Here's how the part is built. I have some questions about the finished solid (model axes, mm). Give positions to 0.01 mm unless a question says otherwise; leave off trailing zeros. Loops run counter-clockwise (first coordinate to the right, second up) from the corner with the lowest first, then second, coordinate; pieces in that order, holes last. Notation, with made-up numbers: M 18.5,86 L 31.5,86 A10 cw 31.5,99 Z; hole C -11.75,71.5 d8. An arc over 180 degrees is marked long. Answer as CSV lines item,"result". Start each with the question number.
Item 1: I want a section at B-B on y = 8.8. List the corners of the cut face in (x, z) for me (3 decimals), plus the area to 4 significant figures.
Item 2: Will these pins go through, and if not, where does the flat tip stop? P1, Ø6.5, axis at x = -3.675, z = 28, coming from the +Y side; P2, Ø5, axis at x = -3.675, z = 7, coming from the +Y side.
Item 3: If we mould it in two halves opening along Y, with no side actions, what happens to faces 1 (the cylindrical face through (9.24, 3.92, 17.74)), 2 (the flat face through (-9.675, 4, 17)), 3 (the cylindrical face through (-6.823, 18.793, 17.745))? For each: released by +Y, released by -Y, zero draft, split by the parting line, or undercut.
Item 4: I want a section at C-C on y = -0.5. List the corners of the cut face in (x, z) for me (3 decimals), plus the area to 3 significant figures.
Item 5: I want a section at A-A on z = 28. List the corners of the cut face in (x, y) for me (3 decimals), plus the area to 3 significant figures.
Item 6: I want a section at D-D on x = -3.5. List the corners of the cut face in (y, z) for me.
Item 7: If I drill on line 1 along X through (y, z) = (3, 7) (3 decimals); line 2 along X through (y, z) = (14.75, 27.5); line 3 along Z through (x, y) = (-2.5, 0.25), over which ranges is the centre line in solid material (lowest first)? Write a range as from..to.
from build123d import *

# Parameters (mm, degrees)
SKETCH1_W           = 40
SKETCH1_H           = 26
BOSS_EXTRUDE1_DEPTH = 35
SKETCH2_R           = 5
CUT_EXTRUDE1_DEPTH  = 45
FILLET1_R           = 10
SKETCH3_R           = 2
CUT_EXTRUDE2_DEPTH  = 26


with BuildPart() as part:
    # Sketch1 → Boss-Extrude1 (new body)
    with BuildSketch(Plane.XY):
        with Locations((10.325, 8.8)):
            Rectangle(SKETCH1_W, SKETCH1_H)
    extrude(amount=BOSS_EXTRUDE1_DEPTH)

    # Sketch2 → Cut-Extrude1 (cut)
    with BuildSketch(Plane.XY.offset(35)):
        with Locations((10.325, 8.8)):
            Circle(SKETCH2_R)
    extrude(amount=-CUT_EXTRUDE1_DEPTH, mode=Mode.SUBTRACT)

    # Fillet1
    fillet1_edges = [part.edges().sort_by_distance(p)[0] for p in [
        (30.325, 21.8, 17.5),
        (-9.675, 21.8, 17.5),
    ]]
    fillet(fillet1_edges, radius=FILLET1_R)

    # Sketch3 → Cut-Extrude2 (cut)
    with BuildSketch(Plane(origin=(0, 21.8, 0), x_dir=(1, 0, 0), z_dir=(0, 1, 0))):
        with Locations(Location((-3.675, -7, 0), (0, 0, 180))):
            Circle(SKETCH3_R)
        with Locations(Location((24.325, -7, 0), (0, 0, 180))):
            Circle(SKETCH3_R)
        with Locations(Location((-3.675, -28, 0), (0, 0, 180))):
            Circle(SKETCH3_R)
        with Locations(Location((24.325, -28, 0), (0, 0, 180))):
            Circle(SKETCH3_R)
    extrude(amount=-CUT_EXTRUDE2_DEPTH, mode=Mode.SUBTRACT)


solid = part.part
Result:
1,outline,"M -9.675,0 L 5.325,0 L 5.325,35 L -9.675,35 Z; M 15.325,0 L 30.325,0 L 30.325,35 L 15.325,35 Z; hole C -3.675,7 d4; hole C -3.675,28 d4; hole C 24.325,7 d4; hole C 24.325,28 d4"
1,area,"1,000 mm^2"
2,P1,"y = 21.77"
2,P2,"y = 21.69"
3,face 1,"undercut"
3,face 2,"zero draft"
3,face 3,"released by +Y"
4,outline,"M -9.675,0 L 30.325,0 L 30.325,35 L -9.675,35 Z; hole C -3.675,7 d4; hole C -3.675,28 d4; hole C 24.325,7 d4; hole C 24.325,28 d4"
4,area,"1,350 mm^2"
5,outline,"M -9.675,-4.2 L -5.675,-4.2 L -5.675,19.8 A10 ccw -9.675,11.8 Z; M -1.675,-4.2 L 22.325,-4.2 L 22.325,21.598 A10 ccw 20.325,21.8 L 0.325,21.8 A10 ccw -1.675,21.598 Z; M 26.325,-4.2 L 30.325,-4.2 L 30.325,11.8 A10 ccw 26.325,19.8 Z; hole C 10.325,8.8 d10"
5,area,"718 mm^2"
6,outline,"M -4.2,0 L 21.04,0 L 21.04,5.01 L -4.2,5.01 Z; M -4.2,8.99 L 21.04,8.99 L 21.04,26.01 L -4.2,26.01 Z; M -4.2,29.99 L 21.04,29.99 L 21.04,35 L -4.2,35 Z"
7,line 1,"-9.675..-5.675, -1.675..22.325, 26.325..30.325"
7,line 2,"-9.23..-5.61, -1.74..22.39, 26.26..29.88"
7,line 3,"0..5.38, 8.62..26.38, 29.62..35"
